CAD build for the part. Positions are in the model's coordinates, mm. Face numbers are marked on the shaded views. A direction names the side the tool comes from. Give positions to 0.01 mm unless a question says otherwise; leave off trailing zeros. Order: outer loops, then holes, each group sorted by start corner. A loop starts at its lowest first (then second) coordinate and runs counter-clockwise, first axis right, second up. Notation, with made-up numbers: M -11.5,16 L 0.5,16 A20 cw 0.5,22 Z; hole C 28,50 d6. An arc over 180 degrees is marked long. Put each result on its own line as item: value. Start each with the question number.
1) Tool access for the marked faces 5 and 6: list every direction of +Z, -Z, +X, -X, +Y, -Y with a clear straight run to the whole face (end or side of a thin tool).
2) Drill centre lines: line 1 (Y direction, x = 0, z = 2); line 2 (Y direction, x = 0, z = 114.5); line 3 (X direction, y = 12, z = 7.5). Where is each one in solid material? Low to high. Write a range as [from, to].
3) Cut at A-A (x = 0). Give the number of separate pieces and of enclosed holes in the cut face, and give its area (3 significant figures).
4) Cut at D-D (z = 115). Write the cut outline in (x, y).
5) Pin check, flat tips, straight feed: pin 1 (5 mm diameter, centred on y = -10, z = 84.5, fed in from -X); pin 2 (6 mm diameter, centred on x = 13.5, z = 98.5, fed in from +Y); pin 3 (8 mm diameter, centred on x = 5, z = 20.5, fed in from -Y). Stop position of each tip, or through.
6) Cut at C-C (z = 22). Write the cut outline in (x, y), and give its area (3 significant figures).
7) Cut at B-B (z = 100). Write the cut outline in (x, y), and give its area (3 significant figures).
8) Two-plate mould, pull along Y, no slides. Class the marked faces 1, 2, 3 and 4: released by +Y, released by -Y, zero draft, split by the parting line, or undercut.
```python
from build123d import *

# Parameters (mm, degrees)
SKETCH1_R            = 32
BODY_DEPTH           = 122
SKETCH2_R            = 20
LIP_BORE_DEPTH       = 122
SKETCH3_R            = 22
BRIDGE_SEAT_DEPTH    = 119
SKETCH4_R            = 25
HOPPER_DEPTH         = 111
SKETCH5_R            = 27
BURR_SEAT_DEPTH      = 50
SKETCH6_R            = 28
PILOT_SEAT_DEPTH     = 30
SKETCH7_R            = 28.46
THREAD_MINOR_DEPTH   = 10
SKETCH8_R            = 29.5
THREAD_RELIEF_DEPTH  = 2
SKETCH9_R            = 33
SKETCH9_R_2          = 30.45
ORING_GROOVE_DEPTH   = 2.7
SKETCH10_R           = 1.65
BURR_SCREW_90_DEPTH  = 6
SKETCH11_R           = 1.65
BURR_SCREW_270_DEPTH = 6
SKETCH12_R           = 1.65
BRIDGE_SCREW_DEPTH   = 11
SKETCH13_R           = 2.5
PLUNGER_HOLE_DEPTH   = 5


with BuildPart() as part:
    # Sketch1 → Body (new body)
    with BuildSketch(Plane.XY):
        with Locations(Location((0, 0, 0), (0, 0, 180))):
            Circle(SKETCH1_R)
    extrude(amount=BODY_DEPTH)

    # Sketch2 → Lip_bore (cut)
    with BuildSketch(Plane.XY):
        with Locations(Location((0, 0, 0), (0, 0, 180))):
            Circle(SKETCH2_R)
    extrude(amount=LIP_BORE_DEPTH, mode=Mode.SUBTRACT)

    # Sketch3 → Bridge_seat (cut)
    with BuildSketch(Plane.XY):
        with Locations(Location((0, 0, 0), (0, 0, 180))):
            Circle(SKETCH3_R)
    extrude(amount=BRIDGE_SEAT_DEPTH, mode=Mode.SUBTRACT)

    # Sketch4 → Hopper (cut)
    with BuildSketch(Plane.XY):
        Circle(SKETCH4_R)
    extrude(amount=HOPPER_DEPTH, mode=Mode.SUBTRACT)

    # Sketch5 → Burr_seat (cut)
    with BuildSketch(Plane.XY):
        Circle(SKETCH5_R)
    extrude(amount=BURR_SEAT_DEPTH, mode=Mode.SUBTRACT)

    # Sketch6 → Pilot_seat (cut)
    with BuildSketch(Plane.XY):
        Circle(SKETCH6_R)
    extrude(amount=PILOT_SEAT_DEPTH, mode=Mode.SUBTRACT)

    # Sketch7 → Thread_minor (cut)
    with BuildSketch(Plane.XY):
        Circle(SKETCH7_R)
    extrude(amount=THREAD_MINOR_DEPTH, mode=Mode.SUBTRACT)

    # Sketch8 → Thread_relief (cut)
    with BuildSketch(Plane.XY.offset(10)):
        Circle(SKETCH8_R)
    extrude(amount=THREAD_RELIEF_DEPTH, mode=Mode.SUBTRACT)

    # Sketch9 → Oring_groove (cut)
    with BuildSketch(Plane.XY.offset(14.65)):
        Circle(SKETCH9_R)
        with Locations(Location((0, 0, 0), (0, 0, 180))):
            Circle(SKETCH9_R_2, mode=Mode.SUBTRACT)
    extrude(amount=ORING_GROOVE_DEPTH, mode=Mode.SUBTRACT)

    # Sketch10 → Burr_screw_90 (cut)
    with BuildSketch(Plane(origin=(0, 26.5, 0), x_dir=(1, 0, 0), z_dir=(0, 1, 0))):
        with Locations(Location((0, -40, 0), (0, 0, 90))):
            Circle(SKETCH10_R)
    extrude(amount=BURR_SCREW_90_DEPTH, mode=Mode.SUBTRACT)

    # Sketch11 → Burr_screw_270 (cut)
    with BuildSketch(Plane(origin=(0, -32.5, 0), x_dir=(1, 0, 0), z_dir=(0, 1, 0))):
        with Locations(Location((0, -40, 0), (0, 0, 90))):
            Circle(SKETCH11_R)
    extrude(amount=BURR_SCREW_270_DEPTH, mode=Mode.SUBTRACT)

    # Sketch12 → Bridge_screw (cut)
    with BuildSketch(Plane(origin=(21.5, 0, 0), x_dir=(0, 0, -1), z_dir=(1, 0, 0))):
        with Locations(Location((-115, 0, 0), (0, 0, 180))):
            Circle(SKETCH12_R)
    extrude(amount=BRIDGE_SCREW_DEPTH, mode=Mode.SUBTRACT)

    # Sketch13 → Plunger_hole (cut)
    with BuildSketch(Plane(origin=(-32.5, 0, 0), x_dir=(0, 0, -1), z_dir=(1, 0, 0))):
        with Locations(Location((-22, 0, 0), (0, 0, 180))):
            Circle(SKETCH13_R)
    extrude(amount=PLUNGER_HOLE_DEPTH, mode=Mode.SUBTRACT)


solid = part.part
```
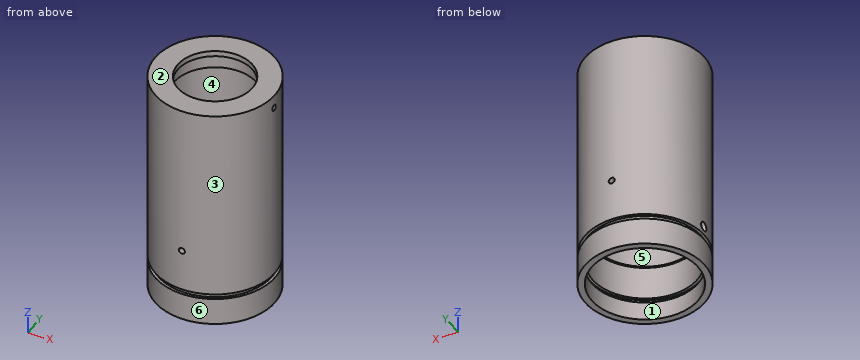
Solution:
1. face 5: -Z
1. face 6: +Z, -Z
2. line 1: [-32, -28.46], [28.46, 32]
2. line 2: [-32, -22], [22, 32]
2. line 3: [-29.66, -25.81], [25.81, 29.66]
3. separate pieces: 4
3. enclosed holes: 0
3. area: 1,470 mm²
4. outline: M 21.94,-1.65 A22 cw long 21.94,1.65 L 31.96,1.65 A32 ccw long 31.96,-1.65 Z
5. pin 1: x = -31.11
5. pin 2: y = 30.23
5. pin 3: y = -31.98
6. outline: M -31.9,-2.5 A32 ccw long -31.9,2.5 L -27.89,2.5 A28 cw long -27.89,-2.5 Z
6. area: 734 mm²
7. outline: C 0,0 d64; hole C 0,0 d50
7. area: 1,250 mm²
8. face 1: undercut
8. face 2: zero draft
8. face 3: split by the parting line
8. face 4: undercut
